```python
from build123d import *

# Parameters (mm, degrees)
F0_R     = 12.7
F1_DEPTH = 25.4
F2_DEPTH = 50.8


with BuildPart() as f1:
    # F0 (on Front) → F1 (new body)
    with BuildSketch(Plane.XZ):
        with BuildLine():
            ThreePointArc((5.042647, -28.126541), (21.916025, -18.336262), (28.575, 0))
            ThreePointArc((28.575, 0), (21.916025, 18.336262), (5.042647, 28.126541))
            ThreePointArc((5.042647, 28.126541), (-28.575, 0), (5.042647, -28.126541))
        make_face()
        with BuildLine():
            ThreePointArc((-11.773215, 4.7625), (0, 12.7), (11.773215, 4.7625))
            Line((11.773215, 4.7625), (19.05, 4.7625))
            Line((19.05, 4.7625), (19.05, -4.7625))
            Line((19.05, -4.7625), (11.773215, -4.7625))
            ThreePointArc((11.773215, -4.7625), (0, -12.7), (-11.773215, -4.7625))
            Line((-11.773215, -4.7625), (-19.05, -4.7625))
            Line((-19.05, -4.7625), (-19.05, 4.7625))
            Line((-19.05, 4.7625), (-11.773215, 4.7625))
        make_face(mode=Mode.SUBTRACT)
        with BuildLine():
            ThreePointArc((-11.773215, -4.7625), (-12.7, 0), (-11.773215, 4.7625))
            Line((-11.773215, 4.7625), (-19.05, 4.7625))
            Line((-19.05, 4.7625), (-19.05, -4.7625))
            Line((-19.05, -4.7625), (-11.773215, -4.7625))
        make_face()
        with BuildLine():
            ThreePointArc((73.025, 0), (68.585683, 12.224174), (57.336765, 18.751028))
            ThreePointArc((57.336765, 18.751028), (34.925, 0), (57.336765, -18.751028))
            ThreePointArc((57.336765, -18.751028), (68.585683, -12.224174), (73.025, 0))
        make_face()
        with Locations((53.975, 0)):
            Circle(F0_R, mode=Mode.SUBTRACT)
        with BuildLine():
            ThreePointArc((5.042647, 28.126541), (21.916025, 18.336262), (28.575, 0))
            ThreePointArc((28.575, 0), (21.916025, -18.336262), (5.042647, -28.126541))
            Line((5.042647, -28.126541), (57.336765, -18.751028))
            ThreePointArc((57.336765, -18.751028), (34.925, 0), (57.336765, 18.751028))
            Line((57.336765, 18.751028), (5.042647, 28.126541))
        make_face()
    extrude(amount=F1_DEPTH)

    # F0 (on Front) → F2 (join)
    with BuildSketch(Plane.XZ):
        with BuildLine():
            ThreePointArc((5.042647, -28.126541), (21.916025, -18.336262), (28.575, 0))
            ThreePointArc((28.575, 0), (21.916025, 18.336262), (5.042647, 28.126541))
            ThreePointArc((5.042647, 28.126541), (-28.575, 0), (5.042647, -28.126541))
        make_face()
        with BuildLine():
            ThreePointArc((-11.773215, 4.7625), (0, 12.7), (11.773215, 4.7625))
            Line((11.773215, 4.7625), (19.05, 4.7625))
            Line((19.05, 4.7625), (19.05, -4.7625))
            Line((19.05, -4.7625), (11.773215, -4.7625))
            ThreePointArc((11.773215, -4.7625), (0, -12.7), (-11.773215, -4.7625))
            Line((-11.773215, -4.7625), (-19.05, -4.7625))
            Line((-19.05, -4.7625), (-19.05, 4.7625))
            Line((-19.05, 4.7625), (-11.773215, 4.7625))
        make_face(mode=Mode.SUBTRACT)
        with BuildLine():
            ThreePointArc((-11.773215, -4.7625), (-12.7, 0), (-11.773215, 4.7625))
            Line((-11.773215, 4.7625), (-19.05, 4.7625))
            Line((-19.05, 4.7625), (-19.05, -4.7625))
            Line((-19.05, -4.7625), (-11.773215, -4.7625))
        make_face()
    extrude(amount=F2_DEPTH)


solid = f1.part
```
Here's how the part is built. I have some questions about the finished solid (model axes, mm). A direction names the side the tool comes from. Round coordinates to 2 decimals unless told otherwise and drop trailing zeros. Order: outer loops, then holes, each group sorted by start corner. A loop starts at its lowest first (then second) coordinate and runs counter-clockwise, first axis right, second up. Notation, with made-up numbers: M 58,79.25 L 68,79.25 A18 ccw 68,109.25 Z; hole C 7.25,-14 d8. An arc over 180 degrees is marked long. Use CSV: the item, a comma, the result in double quotes.
1) On a 3-axis mill with a long thin cutter (end or side, diameter ignored), from which of +Z, -Z, +X, -X, +Y, -Y can I reach the whole of each face in a straight line? I mean faces 5 (the flat face through (22, 0, 0)), 6 (the flat face through (15, -25, 4.762)). Say none if no direction works.
Taken from the geometry:
face 5,"+Z, -Z, +X, -X, +Y"
face 6,"+Y, -Y"
2) I want a section at D-D (z = 11.5). List the corners of the cut face in (x, y) for me, then the cut area to 3 significant figures.
Taken from the geometry:
outline,"M -26.16,-50.8 L -5.39,-50.8 L -5.39,0 L -26.16,0 Z; M 5.39,-50.8 L 26.16,-50.8 L 26.16,-25.4 L 48.59,-25.4 L 48.59,0 L 5.39,0 Z; M 59.36,-25.4 L 69.16,-25.4 L 69.16,0 L 59.36,0 Z"
area,"2,930 mm^2"
3) I want a section at B-B (y = -15). Count the separate pieces of the cut face and the enclosed holes in it, then the cut area to 3 significant figures.
Taken from the geometry:
separate pieces,"1"
enclosed holes,"2"
area,"3,390 mm^2"
4) I'm going to push flat-ended pins straight in: P1, Ø6, axis at y = -31.5, z = -2.5, coming from the +X side (3 decimals); P2, Ø8, axis at x = -11, z = -1, coming from the -Y side; P3, Ø3, axis at y = -40.5, z = 10.5, coming from the -X side; P4, Ø3, axis at x = 59, y = -12, coming from the +Z side. Where does each tip first touch, or does it pass through?
Taken from the geometry:
P1,"x = 28.575"
P2,"y = -50.8"
P3,"x = -27.12"
P4,"z = 18.72"
5) I want a section at A-A (x = 0). List the corners of the cut face in (y, z) for me (3 decimals), then the cut area to 3 significant figures.
Taken from the geometry:
outline,"M -50.8,-28.575 L 0,-28.575 L 0,-12.7 L -50.8,-12.7 Z; M -50.8,12.7 L 0,12.7 L 0,28.575 L -50.8,28.575 Z"
area,"1,610 mm^2"
6) If we mould it in two halves opening along X, with no side actions, what happens to faces 1 (the flat face through (31.556, -12.522, 23.373)), 2 (the cylindrical face through (66.09, -12.52, 3.81)), 3 (the flat face through (15, -25, -4.762)), 4 (the flat face through (39, -25.4, 0))? For each: pulls with the +X half, pulls with the -X half, needs draft (parallel to the pull), parting line crosses it, or undercut.
Taken from the geometry:
face 1,"pulls with the +X half"
face 2,"undercut"
face 3,"undercut"
face 4,"needs draft"
7) I need wall thicknesses on line 1 along Y through (x, z) = (34, -7); line 2 along Z through (x, y) = (-10, -22); line 3 along X through (y, z) = (-38.5, -5). Which ranges of each line are inside material? Lowest first, please. Write a range as [from, to].
Taken from the geometry:
line 1,"[-25.4, 0]"
line 2,"[-26.77, -7.83], [7.83, 26.77]"
line 3,"[-28.13, -11.67], [11.67, 28.13]"
